Part model, mm, in its own coordinate system. A direction names the side the tool comes from. Coordinates: 2 decimals unless noted, no trailing zeros. Write item = value, one per line. Start each with the question number.
Q1. Pull direction Z, two halves, no side cores. Call faces 1 (the flat face through (-4, 0, 15)), 2 (the flat face through (-287, 10, 15)), 3 (the flat face through (-4, 10, 30)): released by +Z, released by -Z, zero draft, split by the parting line, or undercut.
Q2. Pin check, flat tips, straight feed: P1, Ø3, axis at y = 10, z = 8, coming from the +X side; P2, Ø3, axis at y = 9.5, z = 13, coming from the -X side. Stop position of each tip, or through.
Q3. Tool access for faces 4 (the cylindrical face through (-291.06, 11.5, 19.77)), 5 (the flat face through (-4, 10, 0)), 6 (the cylindrical face through (291.06, 11.5, 5.23)): list every direction of +Z, -Z, +X, -X, +Y, -Y with a clear straight run to the whole face (end or side of a thin tool).
Q4. Probe line 1 (X direction, y = 6.5, z = 7); line 2 (X direction, y = 5, z = 7); line 3 (Z direction, x = 274, y = 5.75). List the from-to ranges inside material, lowest first.
from build123d import *

# Parameters (mm, degrees)
SKETCH1_W           = 590
SKETCH1_H           = 20
BOSS_EXTRUDE1_DEPTH = 30
FILLET1_R           = 2
SKETCH6_R           = 5
CUT_EXTRUDE5_DEPTH  = 8
SKETCH7_R           = 5
CUT_EXTRUDE6_DEPTH  = 8
SKETCH8_R           = 3
CUT_EXTRUDE7_DEPTH  = 298.195222034


with BuildPart() as part:
    # Sketch1 → Boss-Extrude1 (new body)
    with BuildSketch(Plane.XY):
        with Locations((0, 10)):
            Rectangle(SKETCH1_W, SKETCH1_H)
    extrude(amount=BOSS_EXTRUDE1_DEPTH)

    # Fillet1
    fillet1_edges = [part.edges().sort_by_distance(p)[0] for p in [
        (295, 10, 30),
        (0, 20, 30),
        (-295, 10, 30),
        (0, 20, 0),
        (295, 10, 0),
        (0, 0, 0),
        (-295, 10, 0),
        (-295, 20, 15),
        (295, 20, 15),
        (295, 0, 15),
        (-295, 0, 15),
        (0, 0, 30),
    ]]
    fillet(fillet1_edges, radius=FILLET1_R)

    # Sketch6 → Cut-Extrude5 (cut)
    with BuildSketch(Plane(origin=(295, 0, 0), x_dir=(0, 0, -1), z_dir=(1, 0, 0))):
        with Locations((-10, 10)):
            Circle(SKETCH6_R)
    extrude(amount=-CUT_EXTRUDE5_DEPTH, mode=Mode.SUBTRACT)

    # Sketch7 → Cut-Extrude6 (cut)
    with BuildSketch(Plane.ZY.offset(295)):
        with Locations((15, 10)):
            Circle(SKETCH7_R)
    extrude(amount=-CUT_EXTRUDE6_DEPTH, mode=Mode.SUBTRACT)

    # Sketch8 → Cut-Extrude7 (cut, through all)
    with BuildSketch(Plane.XZ):
        with Locations(Location((-259, 7, 0), (0, 0, 90))):
            Circle(SKETCH8_R)
        with Locations(Location((274, 7, 0), (0, 0, 270))):
            Circle(SKETCH8_R)
    extrude(amount=-CUT_EXTRUDE7_DEPTH, mode=Mode.SUBTRACT)


solid = part.part
Ans:
q1.face_1 = zero draft
q1.face_2 = undercut
q1.face_3 = released by +Z
q2.P1 = 287
q2.P2 = -287
q3.face_4 = -X
q3.face_5 = -Z, +X, -X, +Y, -Y
q3.face_6 = +X
q4.line_1 = -295 to -262, -256 to 271, 277 to 287
q4.line_2 = -295 to -262, -256 to 271, 277 to 295
q4.line_3 = 0 to 4, 10 to 30
